```python
from build123d import *

# Parameters (mm, degrees)
ESQUISSE1_R        = 2.1
ESQUISSE1_R_2      = 2.5
ESQUISSE1_R_3      = 16.5
ESQUISSE1_R_4      = 7.5
ESQUISSE1_R_5      = 1.5875
ESQUISSE1_W        = 32
ESQUISSE1_H        = 75
BOSS_EXTRU_1_DEPTH = 5


with BuildPart() as part:
    # Esquisse1 → Boss.-Extru.1 (new body)
    with BuildSketch(Plane.XY):
        with BuildLine():
            Line((0, 0), (35, 0))
            Line((35, 0), (35, -5))
            Line((35, -5), (85, -5))
            Line((85, -5), (85, 0))
            Line((85, 0), (98.169872981, 0))
            ThreePointArc((98.169872981, 0), (102.5, 2.641471856), (106.830127019, 0))
            Line((106.830127019, 0), (120, 0))
            Line((120, 0), (120, -5))
            Line((120, -5), (170, -5))
            Line((170, -5), (170, 0.271578296))
            Line((170, 0.271578296), (183.169872981, 0.271578296))
            ThreePointArc((183.169872981, 0.271578296), (187.5, 2.771578296), (191.830127019, 0.271578296))
            Line((191.830127019, 0.271578296), (205, 0.271578296))
            Line((205, 0.271578296), (205, -4.728421704))
            Line((205, -4.728421704), (255, -4.728421704))
            Line((255, -4.728421704), (255, 0.271578296))
            Line((255, 0.271578296), (289.728421704, 0.271578296))
            Line((289.728421704, 0.271578296), (299.227867688, -9.227867688))
            ThreePointArc((299.227867688, -9.227867688), (304.267766953, -10.460654751), (305.500554016, -15.500554016))
            Line((305.500554016, -15.500554016), (315, -25))
            Line((315, -25), (315, -37.898294686))
            ThreePointArc((315, -37.898294686), (317.5, -42.228421704), (315, -46.558548723))
            Line((315, -46.558548723), (315, -59.728421704))
            Line((315, -59.728421704), (310, -59.728421704))
            Line((310, -59.728421704), (310, -109.728421704))
            Line((310, -109.728421704), (315, -109.728421704))
            Line((315, -109.728421704), (315, -149.728421704))
            Line((315, -149.728421704), (310, -149.728421704))
            Line((310, -149.728421704), (310, -199.728421704))
            Line((310, -199.728421704), (315, -199.728421704))
            Line((315, -199.728421704), (315, -212.898294686))
            ThreePointArc((315, -212.898294686), (317.5, -217.228421704), (315, -221.558548723))
            Line((315, -221.558548723), (315, -234.728421704))
            Line((315, -234.728421704), (305.561862178, -244.166559526))
            ThreePointArc((305.561862178, -244.166559526), (304.267766953, -248.996188657), (299.438137822, -250.290283883))
            Line((299.438137822, -250.290283883), (290, -259.728421704))
            Line((290, -259.728421704), (255, -259.728421704))
            Line((255, -259.728421704), (255, -254.728421704))
            Line((255, -254.728421704), (205, -254.728421704))
            Line((205, -254.728421704), (205, -259.728421704))
            Line((205, -259.728421704), (191.830127019, -259.728421704))
            ThreePointArc((191.830127019, -259.728421704), (187.5, -262.228421704), (183.169872981, -259.728421704))
            Line((183.169872981, -259.728421704), (170, -259.728421704))
            Line((170, -259.728421704), (170, -254.728421704))
            Line((170, -254.728421704), (120, -254.728421704))
            Line((120, -254.728421704), (120, -259.728421704))
            Line((120, -259.728421704), (106.830127019, -259.728421704))
            ThreePointArc((106.830127019, -259.728421704), (102.5, -262.228421704), (98.169872981, -259.728421704))
            Line((98.169872981, -259.728421704), (85, -259.728421704))
            Line((85, -259.728421704), (85, -254.728421704))
            Line((85, -254.728421704), (35, -254.728421704))
            Line((35, -254.728421704), (35, -259.728421704))
            Line((35, -259.728421704), (0, -259.728421704))
            Line((0, -259.728421704), (-9.438137822, -250.290283883))
            ThreePointArc((-9.438137822, -250.290283883), (-14.267766953, -248.996188657), (-15.561862178, -244.166559526))
            Line((-15.561862178, -244.166559526), (-25, -234.728421704))
            Line((-25, -234.728421704), (-25, -221.558548723))
            ThreePointArc((-25, -221.558548723), (-27.5, -217.228421704), (-25, -212.898294686))
            Line((-25, -212.898294686), (-25, -199.728421704))
            Line((-25, -199.728421704), (-20, -199.728421704))
            Line((-20, -199.728421704), (-20, -149.728421704))
            Line((-20, -149.728421704), (-25, -149.728421704))
            Line((-25, -149.728421704), (-25, -110))
            Line((-25, -110), (-20, -110))
            Line((-20, -110), (-20, -60))
            Line((-20, -60), (-25, -60))
            Line((-25, -60), (-25, -46.558548723))
            ThreePointArc((-25, -46.558548723), (-27.5, -42.228421704), (-25, -37.898294686))
            Line((-25, -37.898294686), (-25, -25))
            Line((-25, -25), (-15.500554016, -15.500554016))
            ThreePointArc((-15.500554016, -15.500554016), (-14.267766953, -10.460654751), (-9.227867688, -9.227867688))
            Line((-9.227867688, -9.227867688), (0, 0))
        make_face()
        with Locations((102.5, -257.228421704)):
            Circle(ESQUISSE1_R, mode=Mode.SUBTRACT)
        with Locations(Location((187.5, -257.228421704, 0), (0, 0, 180))):
            Circle(ESQUISSE1_R, mode=Mode.SUBTRACT)
        with Locations(Location((102.5, -2.228421704, 0), (0, 0, 180))):
            Circle(ESQUISSE1_R, mode=Mode.SUBTRACT)
        with Locations((187.5, -2.228421704)):
            Circle(ESQUISSE1_R, mode=Mode.SUBTRACT)
        with Locations((-10.732233047, -13.996188657)):
            Circle(ESQUISSE1_R, mode=Mode.SUBTRACT)
        with Locations(Location((300.732233047, -13.996188657, 0), (0, 0, 180))):
            Circle(ESQUISSE1_R, mode=Mode.SUBTRACT)
        with Locations((300.732233047, -245.460654751)):
            Circle(ESQUISSE1_R, mode=Mode.SUBTRACT)
        with Locations(Location((-10.732233047, -245.460654751, 0), (0, 0, 180))):
            Circle(ESQUISSE1_R, mode=Mode.SUBTRACT)
        with Locations((-22.5, -217.228421704)):
            Circle(ESQUISSE1_R, mode=Mode.SUBTRACT)
        with Locations(Location((-22.5, -42.228421704, 0), (0, 0, 180))):
            Circle(ESQUISSE1_R, mode=Mode.SUBTRACT)
        with Locations((312.5, -42.228421704)):
            Circle(ESQUISSE1_R, mode=Mode.SUBTRACT)
        with Locations(Location((312.5, -217.228421704, 0), (0, 0, 180))):
            Circle(ESQUISSE1_R, mode=Mode.SUBTRACT)
        with Locations(Location((300.5, -155.228421704, 0), (0, 0, 180))):
            Circle(ESQUISSE1_R_2, mode=Mode.SUBTRACT)
        with Locations(Location((300.5, -104.228421704, 0), (0, 0, 180))):
            Circle(ESQUISSE1_R_2, mode=Mode.SUBTRACT)
        with Locations((145, -35)):
            Circle(ESQUISSE1_R_3, mode=Mode.SUBTRACT)
        with Locations((145, -129.864210852)):
            Circle(ESQUISSE1_R_4, mode=Mode.SUBTRACT)
        with Locations(Location((292.5, -104.228421704, 0), (0, 0, 180))):
            Circle(ESQUISSE1_R_2, mode=Mode.SUBTRACT)
        with Locations(Location((292.5, -155.228421704, 0), (0, 0, 180))):
            Circle(ESQUISSE1_R_2, mode=Mode.SUBTRACT)
        with Locations(Location((284.5, -104.228421704, 0), (0, 0, 180))):
            Circle(ESQUISSE1_R_2, mode=Mode.SUBTRACT)
        with Locations(Location((284.5, -155.228421704, 0), (0, 0, 180))):
            Circle(ESQUISSE1_R_2, mode=Mode.SUBTRACT)
        with Locations((-10.5, -104.228421704)):
            Circle(ESQUISSE1_R_2, mode=Mode.SUBTRACT)
        with Locations((-2.5, -104.228421704)):
            Circle(ESQUISSE1_R_2, mode=Mode.SUBTRACT)
        with Locations((5.5, -104.228421704)):
            Circle(ESQUISSE1_R_2, mode=Mode.SUBTRACT)
        with Locations((-10.5, -155.228421704)):
            Circle(ESQUISSE1_R_2, mode=Mode.SUBTRACT)
        with Locations((-2.5, -155.228421704)):
            Circle(ESQUISSE1_R_2, mode=Mode.SUBTRACT)
        with Locations((5.5, -155.228421704)):
            Circle(ESQUISSE1_R_2, mode=Mode.SUBTRACT)
        with Locations(Location((145, -224.728421704, 0), (0, 0, 180))):
            Circle(ESQUISSE1_R_3, mode=Mode.SUBTRACT)
        with Locations((91.471682341, -119.185385667)):
            Circle(ESQUISSE1_R_5, mode=Mode.SUBTRACT)
        with Locations((104.171682341, -119.185385667)):
            Circle(ESQUISSE1_R_5, mode=Mode.SUBTRACT)
        with Locations((97.821682341, -119.185385667)):
            Circle(ESQUISSE1_R_5, mode=Mode.SUBTRACT)
        with Locations((110.521682341, -119.185385667)):
            Circle(ESQUISSE1_R_5, mode=Mode.SUBTRACT)
        with Locations((116.871682341, -119.185385667)):
            Circle(ESQUISSE1_R_5, mode=Mode.SUBTRACT)
        with Locations((129.571682341, -119.185385667)):
            Circle(ESQUISSE1_R_5, mode=Mode.SUBTRACT)
        with Locations((123.221682341, -119.185385667)):
            Circle(ESQUISSE1_R_5, mode=Mode.SUBTRACT)
        with Locations((129.571682341, -150.427385667)):
            Circle(ESQUISSE1_R_5, mode=Mode.SUBTRACT)
        with Locations((123.221682341, -150.427385667)):
            Circle(ESQUISSE1_R_5, mode=Mode.SUBTRACT)
        with Locations((116.871682341, -150.427385667)):
            Circle(ESQUISSE1_R_5, mode=Mode.SUBTRACT)
        with Locations((110.521682341, -150.427385667)):
            Circle(ESQUISSE1_R_5, mode=Mode.SUBTRACT)
        with Locations((104.171682341, -150.427385667)):
            Circle(ESQUISSE1_R_5, mode=Mode.SUBTRACT)
        with Locations((97.821682341, -150.427385667)):
            Circle(ESQUISSE1_R_5, mode=Mode.SUBTRACT)
        with Locations((91.471682341, -150.427385667)):
            Circle(ESQUISSE1_R_5, mode=Mode.SUBTRACT)
        with Locations(Location((198.528317659, -119.185385667, 0), (0, 0, 180))):
            Circle(ESQUISSE1_R_5, mode=Mode.SUBTRACT)
        with Locations(Location((192.178317659, -119.185385667, 0), (0, 0, 180))):
            Circle(ESQUISSE1_R_5, mode=Mode.SUBTRACT)
        with Locations(Location((185.828317659, -119.185385667, 0), (0, 0, 180))):
            Circle(ESQUISSE1_R_5, mode=Mode.SUBTRACT)
        with Locations(Location((179.478317659, -119.185385667, 0), (0, 0, 180))):
            Circle(ESQUISSE1_R_5, mode=Mode.SUBTRACT)
        with Locations(Location((173.128317659, -119.185385667, 0), (0, 0, 180))):
            Circle(ESQUISSE1_R_5, mode=Mode.SUBTRACT)
        with Locations(Location((166.778317659, -119.185385667, 0), (0, 0, 180))):
            Circle(ESQUISSE1_R_5, mode=Mode.SUBTRACT)
        with Locations(Location((160.428317659, -119.185385667, 0), (0, 0, 180))):
            Circle(ESQUISSE1_R_5, mode=Mode.SUBTRACT)
        with Locations(Location((160.428317659, -150.427385667, 0), (0, 0, 180))):
            Circle(ESQUISSE1_R_5, mode=Mode.SUBTRACT)
        with Locations(Location((166.778317659, -150.427385667, 0), (0, 0, 180))):
            Circle(ESQUISSE1_R_5, mode=Mode.SUBTRACT)
        with Locations(Location((173.128317659, -150.427385667, 0), (0, 0, 180))):
            Circle(ESQUISSE1_R_5, mode=Mode.SUBTRACT)
        with Locations(Location((179.478317659, -150.427385667, 0), (0, 0, 180))):
            Circle(ESQUISSE1_R_5, mode=Mode.SUBTRACT)
        with Locations(Location((185.828317659, -150.427385667, 0), (0, 0, 180))):
            Circle(ESQUISSE1_R_5, mode=Mode.SUBTRACT)
        with Locations(Location((192.178317659, -150.427385667, 0), (0, 0, 180))):
            Circle(ESQUISSE1_R_5, mode=Mode.SUBTRACT)
        with Locations(Location((198.528317659, -150.427385667, 0), (0, 0, 180))):
            Circle(ESQUISSE1_R_5, mode=Mode.SUBTRACT)
        with Locations((231, -130)):
            Rectangle(ESQUISSE1_W, ESQUISSE1_H, mode=Mode.SUBTRACT)
        with Locations((59, -130)):
            Rectangle(ESQUISSE1_W, ESQUISSE1_H, mode=Mode.SUBTRACT)
    extrude(amount=BOSS_EXTRU_1_DEPTH)


solid = part.part
```
Here's how the part is built. I have some questions about the finished solid (model axes, mm). Give positions to 0.01 mm unless a question says otherwise; leave off trailing zeros. Order: outer loops, then holes, each group sorted by start corner. A loop starts at its lowest first (then second) coordinate and runs counter-clockwise, first axis right, second up. Notation, with made-up numbers: M 15,-38 L 25,-38 A10 ccw 25,-25 Z; hole C 60.25,47.25 d4. An arc over 180 degrees is marked long. Use a Markdown table: item, result. Add a question column.
1. Suppose I cut it at D-D (z = 1.05). Give the number of separate pieces and of enclosed holes in the cut face, and give its area (3 significant figures).
2. For pin 1 Ø1.5 at (x, z) = (24, 3.5) entering from -Y; pin 2 Ø1.5 at (y, z) = (-225.5, 2) entering from +X; pin 3 Ø1.5 at (y, z) = (-166, 3.5) entering from -X, each with a flat end and sliding along its axis, tell me the tip position at first contact or that it passes through.
3. I need wall thicknesses on probe 1 along Y at (x, z) = (5.5, 2.7); probe 2 along X at (y, z) = (-93, 1.9); probe 3 along X at (y, z) = (-129.5, 3.85). Which ranges of each line are inside material? Lowest first, please. Write a range as from..to.
4. Suppose I cut it at B-B (x = 20). List the corners of the cut face in (y, z) for me, and give its area (3 significant figures).
5. If we mould it in two halves opening along X, with no side actions, what happens to faces 1 (the flat face through (-20, -20, 2)), 2 (the cylindrical face through (128.516, -34.275, 2.465)), 3 (the flat face through (147, -98, 0))? For each: +X half, -X half, draft (parallel to the pull), parting line (faces both ways), or undercut.
6. Suppose I cut it at A-A (x = 145). List the corners of the cut face in (y, z) for me.
7. Suppose I cut it at C-C (y = -192). List the corners of the cut face in (x, z) for me, and give its area (3 significant figures).
Results list:
| question | item | result |
|---|---|---|
| 1 | separate pieces | 1 |
| 1 | enclosed holes | 57 |
| 1 | area | 77,500 mm² |
| 2 | pin 1 | stops at y = -259.73 |
| 2 | pin 2 | stops at x = 315 |
| 2 | pin 3 | stops at x = -20 |
| 3 | probe 1 | y = -259.73..-157.73, -152.73..-106.73, -101.73..0 |
| 3 | probe 2 | x = -20..43, 75..215, 247..310 |
| 3 | probe 3 | x = -25..43, 75..137.51, 152.49..215, 247..315 |
| 4 | outline | M -259.73,0 L 0,0 L 0,5 L -259.73,5 Z |
| 4 | area | 1,300 mm² |
| 5 | face 1 | -X half |
| 5 | face 2 | undercut |
| 5 | face 3 | draft |
| 6 | outline | M -254.73,0 L -241.23,0 L -241.23,5 L -254.73,5 Z; M -208.23,0 L -137.36,0 L -137.36,5 L -208.23,5 Z; M -122.36,0 L -51.5,0 L -51.5,5 L -122.36,5 Z; M -18.5,0 L -5,0 L -5,5 L -18.5,5 Z |
| 7 | outline | M -20,0 L 310,0 L 310,5 L -20,5 Z |
| 7 | area | 1,650 mm² |
